Geometry check sheet. Reference: the model listing, model coordinates, mm. A direction names the side the tool comes from. Coordinates: 2 decimals unless noted, no trailing zeros. Write each loop counter-clockwise with the first axis right and the second up, starting at its lowest first coordinate (ties: lowest second). Pieces come first, ordered by that corner, then holes. Notation, with made-up numbers: M -28,-20 L 18,-20 A34 ccw 18,10 Z; hole C 0.5,79 d6. An arc over 180 degrees is marked long. Put each result on its own line as item: value. Start each with the question number.
1) Mould release check, pull along Y, two halves, no side actions. Record for faces 3 (the flat face through (-179, 0, -6)), 4 (the flat face through (-313.97, 75.99, 2.03)): released by +Y, released by -Y, zero draft, split by the parting line, or undercut.
2) Gauge pin test, flat ends, axial feed: pin 1 (0.8 mm diameter, centred on x = -318.5, z = 6, fed in from +Y); pin 2 (10 mm diameter, centred on y = 54.5, z = 4.5, fed in from +X); pin 3 (4 mm diameter, centred on x = -89, y = 57.5, fed in from +Z); pin 4 (10 mm diameter, centred on x = -77, y = 16, fed in from -Z). Record the tip position at first contact, or that the pin passes through.
3) Scan lines: line 1 along Y through (x, z) = (-128.5, -27.5); line 2 along Z through (x, y) = (-70, 37); line 3 along Z through (x, y) = (-309, 110). Record each from-to range of solid material in increasing order.
4) Set-up check for faces 1 (the flat face through (-305.642, 75.994, -7.904)), 2 (the flat face through (-152, 141.943, -8)): record each of +Z, -Z, +X, -X, +Y, -Y from which the full face is reachable in a straight line by a thin tool's end or side.
5) Cross-section at A-A on x = -134. Record the cut outline in (y, z).
from build123d import *

# Parameters (mm, degrees)
EXTRUDE_THIN1_DEPTH   = 150
SKETCH5_W             = 290.970262873
SKETCH5_H             = 4
EXTRUDE_THIN2_DEPTH   = 42
EXTRUDE_THIN2_2_DEPTH = 42
FILLET6_R             = 40
EXTRUDE_THIN7_DEPTH   = 146
FILLET14_R            = 40
SKETCH25_W            = 46
SKETCH25_H            = 150
BOSS_EXTRUDE1_DEPTH   = 2
FILLET22_R            = 30
FILLET28_R            = 30
FILLET32_R            = 20
SKETCH29_W            = 6.511049677
SKETCH29_H            = 4.056851241
BOSS_EXTRUDE2_DEPTH   = 42
EXTRUDE_THIN8_DEPTH   = 142


with BuildPart() as part:
    # Sketch2 → Extrude-Thin1 (new body)
    with BuildSketch(Plane(origin=(0, 0, 0), x_dir=(1, 0, 0), z_dir=(0, 1, 0))):
        Polygon((-30.965120595, -2.565260163), (-320.965120595, -26.307498403), (-320.801927023, -28.300829248), (-30.801927023, -4.558591008), align=None)
    extrude(amount=EXTRUDE_THIN1_DEPTH)



with BuildPart() as body_2:
    # Sketch5 → Extrude-Thin2 (new body)
    with BuildSketch(Plane(origin=(0.002452129, 0, 0.029951579), x_dir=(-0.9966654225627806, 0, 0.08159678589107741), z_dir=(-0.08159678589107741, 0, -0.9966654225627806))):
        with Locations((176.556313424, 2)):
            Rectangle(SKETCH5_W, SKETCH5_H)
    extrude(amount=EXTRUDE_THIN2_DEPTH)

    # Fillet14
    fillet14_edges = [body_2.edges().sort_by_distance(p)[0] for p in [
        (-324.392185602, 2, -15.552449344),
    ]]
    fillet(fillet14_edges, radius=FILLET14_R)


with BuildPart() as body_3:
    # Sketch5 → Extrude-Thin2 2 (new body)
    with BuildSketch(Plane(origin=(0.002452129, 0, 0.029951579), x_dir=(-0.9966654225627806, 0, 0.08159678589107741), z_dir=(-0.08159678589107741, 0, -0.9966654225627806))):
        with Locations((176.556313424, 148)):
            Rectangle(SKETCH5_W, SKETCH5_H)
    extrude(amount=EXTRUDE_THIN2_2_DEPTH)

    # Fillet6
    fillet6_edges = [body_3.edges().sort_by_distance(p)[0] for p in [
        (-324.392185602, 148, -15.552449344),
    ]]
    fillet(fillet6_edges, radius=FILLET6_R)


with BuildPart() as part_1:
    add(part.part)

    add(body_3.part)  # Extrude-Thin7 merges body 3
    # Sketch11 → Extrude-Thin7 (add)
    with BuildSketch(Plane.XZ.offset(-146)):
        Polygon((-278.003111059, -19.350312998), (-281.936630301, -19.587972456), (-284.5255687, -18.81632078), (-290.805852057, -18.238730686), (-291.798277728, -17.537013607), (-298.288108084, -15.145025876), (-304.254167802, -11.68113065), (-309.528907685, -7.251025667), (-313.810104121, -2.200536359), (-317.466443209, 4.043933459), (-318.345283528, 5.696861164), (-319.86163909, 10.560086826), (-321.089242867, 17.33995769), (-321.128314167, 24.314167558), (-320.965120595, 26.307498403), (-318.97178975, 26.144304832), (-319.127856228, 24.238027995), (-319.090248803, 17.52511906), (-317.915603526, 11.037730019), (-316.491598121, 6.470687959), (-315.719800302, 5.019086377), (-312.17205348, -1.039924404), (-308.112866331, -5.828511332), (-303.100359764, -10.038373964), (-297.433799934, -13.328379507), (-290.85904721, -15.751667479), (-290.088883869, -16.296228937), (-284.144627091, -16.842915072), (-281.704255181, -17.570285439), (-278.123729185, -17.353953494), align=None)
    extrude(amount=EXTRUDE_THIN7_DEPTH)


    add(body_2.part)  # Boss-Extrude1 merges body 2
    # Sketch25 → Boss-Extrude1 (add)
    with BuildSketch(Plane(origin=(-30.967572724, 0, 2.535308584), x_dir=(-0.08159678589107766, 0, -0.9966654225627805), z_dir=(0.9966654225627803, 0, -0.08159678589107765))):
        with Locations((20.969948211, 75)):
            Rectangle(SKETCH25_W, SKETCH25_H)
    extrude(amount=BOSS_EXTRUDE1_DEPTH)

    # Fillet22
    fillet22_edges = [part_1.edges().sort_by_distance(p)[0] for p in [
        (-30.965120595, 75, 2.565260163),
    ]]
    fillet(fillet22_edges, radius=FILLET22_R)

    # Fillet28
    fillet28_edges = [part_1.edges().sort_by_distance(p)[0] for p in [
        (-28.808596178, 75, 4.395397436),
    ]]
    fillet(fillet28_edges, radius=FILLET28_R)

    # Fillet32
    # the kernel refuses this fillet: 20 mm, written as the material it takes off along each edge
    with BuildSketch(Plane(origin=(-32.562048329, -21.794494718, -41.451212002), x_dir=(0.08159678589107701, 0, 0.9966654225627805), z_dir=(0, 1, 0))) as fillet32_piece_1:
        with BuildLine():
            CenterArc((8.717797887, -20), FILLET32_R, 90, 25.841932763)
            Line((0, -2), (0, 0))
            Line((0, 0), (8.717797887, 0))
        make_face()
    extrude(amount=193.588989435, mode=Mode.SUBTRACT)

    # Sketch29 → Boss-Extrude2 (add)
    with BuildSketch(Plane(origin=(0.002452129, 0, 0.029951579), x_dir=(-0.9966654225627805, 0, 0.0815967858910774), z_dir=(-0.0815967858910774, 0, -0.9966654225627805))):
        with Locations((150.499315868, 143.971574379)):
            Rectangle(SKETCH29_W, SKETCH29_H)
    extrude(amount=BOSS_EXTRUDE2_DEPTH)

    # Sketch35 → Extrude-Thin8 (add)
    with BuildSketch(Plane.XZ.offset(-146)):
        Polygon((-34.392185602, -39.294687585), (-38.941474001, -38.922238312), (-38.77828043, -36.928907467), (-34.228992031, -37.30135674), align=None)
    extrude(amount=EXTRUDE_THIN8_DEPTH)


solid = part_1.part
Answer key:
1. face 3: released by -Y
1. face 4: undercut
2. pin 1: stops at y = 150
2. pin 2: stops at x = -41.38
2. pin 3: stops at z = 9.49
2. pin 4: stops at z = 5.92
3. line 1: y = 0 to 4, 146 to 150
3. line 2: z = 5.76 to 7.77
3. line 3: z = -7.7 to -4.78, 25.33 to 27.33
4. face 1: none
4. face 2: -Z
5. outline: M 0,-31.14 L 4,-31.14 L 4,11 L 146,11 L 146,-31.14 L 150,-31.14 L 150,13.01 L 0,13.01 Z
